from build123d import *

# Parameters (mm, degrees)
SKETCH_4_W               = 40
SKETCH_4_H               = 40
EXTRUDE_1_DEPTH          = 10
SKETCH_1_R               = 5
CUT_EXTRUDE_1_DEPTH      = 19
SKETCH_5_W               = 40
SKETCH_5_H               = 10
EXTRUDE_2_DEPTH          = 55
SKETCH_6_W               = 40
SKETCH_6_H               = 10
EXTRUDE_3_DEPTH          = 97
SKETCH_7_R               = 1.5
CUT_EXTRUDE_2_DEPTH      = 17
PATTERN_LINEAR_1_COUNT   = 2
PATTERN_LINEAR_1_PITCH   = 10
SKETCH_10_R              = 1
EXTRUDE_5_DEPTH          = 2
PATTERN_CIRCULAR_3_COUNT = 4
DRAFT_2_ANGLE            = 15
DRAFT_3_ANGLE            = 15
DRAFT_4_ANGLE            = 15
DRAFT_5_ANGLE            = 15


with BuildPart() as part:
    # Sketch 4 → Extrude 1 (new body)
    with BuildSketch(Plane.XY):
        Rectangle(SKETCH_4_W, SKETCH_4_H)
    extrude(amount=EXTRUDE_1_DEPTH)

    # Sketch 1 → Cut-Extrude 1 (cut)
    with BuildSketch(Plane.XY):
        Circle(SKETCH_1_R)
    extrude(amount=CUT_EXTRUDE_1_DEPTH, mode=Mode.SUBTRACT)

    # Sketch 5 → Extrude 2 (add)
    with BuildSketch(Plane(origin=(0, 20, 0), x_dir=(1, 0, 0), z_dir=(0, 1, 0))):
        with Locations((0, -5)):
            Rectangle(SKETCH_5_W, SKETCH_5_H)
    extrude(amount=EXTRUDE_2_DEPTH)

    # Sketch 6 → Extrude 3 (add)
    with BuildSketch(Plane.XY.offset(10)):
        with Locations((0, 70)):
            Rectangle(SKETCH_6_W, SKETCH_6_H)
    extrude(amount=EXTRUDE_3_DEPTH)

    # Sketch 7 → Cut-Extrude 2 (cut)
    with BuildSketch(Plane(origin=(0, 75, 0), x_dir=(1, 0, 0), z_dir=(0, 1, 0))):
        with Locations(Location((0, -45.729405638, 0), (0, 0, 180))):
            Circle(SKETCH_7_R)
    cut_extrude_2 = extrude(amount=-CUT_EXTRUDE_2_DEPTH, mode=Mode.SUBTRACT)

    # Pattern Linear 1: Cut-Extrude 2 ×2
    with Locations(*[(-i * PATTERN_LINEAR_1_PITCH, 0, 0) for i in range(1, PATTERN_LINEAR_1_COUNT)]):
        add(cut_extrude_2, mode=Mode.SUBTRACT)

    # Sketch 10 → Extrude 5 (add)
    with BuildSketch(Plane.XY):
        with Locations((0, -10.379430626)):
            Circle(SKETCH_10_R)
    extrude_5 = extrude(amount=-EXTRUDE_5_DEPTH)

    # Pattern Circular 3: Extrude 5 ×4 about axis
    pattern_circular_3_axis = Axis((0, 0, 0), (0, 0, 1))
    for i in range(1, PATTERN_CIRCULAR_3_COUNT):
        add(extrude_5.rotate(pattern_circular_3_axis, i * 360 / PATTERN_CIRCULAR_3_COUNT))

    # Draft 2
    draft_2_faces = [part.faces().sort_by_distance(p)[0] for p in [
        (-1, -10.379430626, -1),
    ]]
    draft(draft_2_faces, Plane(origin=(0, -10.379430626, -2), x_dir=(-1, 0, 0), z_dir=(0, 0, -1)), DRAFT_2_ANGLE)

    # Draft 3
    draft_3_faces = [part.faces().sort_by_distance(p)[0] for p in [
        (10.379430626, -1, -1),
    ]]
    draft(draft_3_faces, Plane(origin=(10.379430626, 0, -2), x_dir=(-1, 0, 0), z_dir=(0, 0, -1)), DRAFT_3_ANGLE)

    # Draft 4
    draft_4_faces = [part.faces().sort_by_distance(p)[0] for p in [
        (1, 10.379430626, -1),
    ]]
    draft(draft_4_faces, Plane(origin=(0, 10.379430626, -2), x_dir=(-1, 0, 0), z_dir=(0, 0, -1)), DRAFT_4_ANGLE)

    # Draft 5
    draft_5_faces = [part.faces().sort_by_distance(p)[0] for p in [
        (-10.379430626, 1, -1),
    ]]
    draft(draft_5_faces, Plane(origin=(-10.379430626, 0, -2), x_dir=(-1, 0, 0), z_dir=(0, 0, -1)), DRAFT_5_ANGLE)


solid = part.part
Can you work these out from the model? Positions are in its coordinate system, mm. A direction names the side the tool comes from. Coordinates: 2 decimals unless noted, no trailing zeros. Write each loop counter-clockwise with the first axis right and the second up, starting at its lowest first coordinate (ties: lowest second). Pieces come first, ordered by that corner, then holes. Notation, with made-up numbers: (83.25, -10) -> (103.25, -10) arc R9 cw to (103.25, 0) -> close; hole circle Ø3 at (12, -31.75). An arc over 180 degrees is marked (long way). Write item = value, one per line.
(1) Thinking about a two-plate mould opening in X: for faces 3 (the face through (0.652, -9.357, -1.208)), 4 (the face through (0.195, 70.07, 47.217)), 5 (the face through (-20, 66, 33)), which applies, +X half, -X half, draft (parallel to the pull), parting line (faces both ways), or undercut?
Verdict:
face_3 = parting line
face_4 = undercut
face_5 = -X half
(2) For pin 1 (1.8 mm diameter, centred on x = 0, z = 45.73, fed in from +Y); pin 2 (12 mm diameter, centred on x = 9.5, y = 42, fed in from -Z); pin 3 (4 mm diameter, centred on x = -4, y = 32.5, fed in from +Z); pin 4 (2 mm diameter, centred on x = 14.5, z = 92, fed in from -Y), each with a flat end and sliding along its axis, tell me the tip position at first contact or that it passes through.
Verdict:
pin_1 = through
pin_2 = 0
pin_3 = 10
pin_4 = 65
(3) Imagine slicing it at A-A (z = 83.5). Please give me the cut outline in (x, y).
Verdict:
outline = (-20, 65) -> (20, 65) -> (20, 75) -> (-20, 75) -> close
(4) Imagine slicing it at B-B (x = 15.5). Please give me the cut outline in (y, z).
Verdict:
outline = (-20, 0) -> (75, 0) -> (75, 107) -> (65, 107) -> (65, 10) -> (-20, 10) -> close
(5) On a 3-axis mill with a long thin cutter (end or side, diameter ignored), from which of +Z, -Z, +X, -X, +Y, -Y can I reach the whole of each face in a straight line? I mean faces 1 (the face through (0, 65, 58)), 2 (the face through (0, 70, 107)). Say none if no direction works.
Verdict:
face_1 = +Z, +X, -X, -Y
face_2 = +Z, +X, -X, +Y, -Y
(6) If I drill on probe 1 along Z at (x, y) = (-10, 70.75); probe 2 along Y at (x, z) = (0, 6.25); probe 3 along Z at (x, y) = (-14, 67), over which ranges is the centre line in solid material (lowest first)?
Verdict:
probe_1 = 0 to 44.23, 47.23 to 107
probe_2 = -20 to -5, 5 to 75
probe_3 = 0 to 107
(7) Imagine slicing it at C-C (y = 39). Please give me the cut outline in (x, z).
Verdict:
outline = (-20, 0) -> (20, 0) -> (20, 10) -> (-20, 10) -> close
